```python
from build123d import *

# Parameters (mm, degrees)
BOSS_EXTRUDE1_DEPTH                   = 3.175
F_10_0_1935_DIAMETER_HOLE1_AT_2_COUNT = 2
F_10_0_1935_DIAMETER_HOLE1_AT_2_PITCH = 25.4
F_10_0_1935_DIAMETER_HOLE1_AT_3_COUNT = 2
F_10_0_1935_DIAMETER_HOLE1_AT_3_PITCH = 28.398063314
F_10_0_1935_DIAMETER_HOLE1_AT_4_COUNT = 2
F_10_0_1935_DIAMETER_HOLE1_AT_4_PITCH = 52.363441445


with BuildPart() as part:
    # Sketch2 → Boss-Extrude1 (new body)
    with BuildSketch(Plane(origin=(0, 0, 0), x_dir=(1, 0, 0), z_dir=(0, 1, 0))):
        Polygon((-0.378728756, 269.21115375), (50.421271244, 269.21115375), (50.421271244, 243.81115375), (37.721271244, 193.01115375), (12.321271244, 193.01115375), (-0.378728756, 243.81115375), align=None)
    extrude(amount=BOSS_EXTRUDE1_DEPTH)

    # Sketch7 → #10 (0.1935) Diameter Hole1 (revolve, cut)
    with BuildSketch(Plane(origin=(37.721271244, 0, -256.51115375), x_dir=(0, 0, -1), z_dir=(1, 0, 0))):
        Polygon((0, 0), (0, 3.175), (2.45745, 3.175), (2.45745, 3.177605133), (5.2197, 0), align=None)
    f_10_0_1935_diameter_hole1 = revolve(axis=Axis((37.721271244, -6.35, -256.51115375), (0, 1, 0)), mode=Mode.SUBTRACT)

    # #10 (0.1935) Diameter Hole1 at 2: #10 (0.1935) Diameter Hole1 ×2
    with Locations(*[(-i * F_10_0_1935_DIAMETER_HOLE1_AT_2_PITCH, 0, 0) for i in range(1, F_10_0_1935_DIAMETER_HOLE1_AT_2_COUNT)]):
        add(f_10_0_1935_diameter_hole1, mode=Mode.SUBTRACT)

    # #10 (0.1935) Diameter Hole1 at 3: #10 (0.1935) Diameter Hole1 ×2
    with Locations(*[Vector(-0.44721359549995443, 0, 0.8944271909999176) * (i * F_10_0_1935_DIAMETER_HOLE1_AT_3_PITCH) for i in range(1, F_10_0_1935_DIAMETER_HOLE1_AT_3_COUNT)]):
        add(f_10_0_1935_diameter_hole1, mode=Mode.SUBTRACT)

    # #10 (0.1935) Diameter Hole1 at 4: #10 (0.1935) Diameter Hole1 ×2
    with Locations(*[Vector(-0.24253562503633175, 0, 0.9701425001453322) * (i * F_10_0_1935_DIAMETER_HOLE1_AT_4_PITCH) for i in range(1, F_10_0_1935_DIAMETER_HOLE1_AT_4_COUNT)]):
        add(f_10_0_1935_diameter_hole1, mode=Mode.SUBTRACT)


solid = part.part
```
Geometry check sheet. Reference: the model listing, model coordinates, mm. Give positions to 0.01 mm unless a question says otherwise; leave off trailing zeros. Loops run counter-clockwise (first coordinate to the right, second up) from the corner with the lowest first, then second, coordinate; pieces in that order, holes last. Notation, with made-up numbers: M -23,-38 L 20,-38 A31 ccw 20,-4 Z; hole C 53.25,83.5 d10. An arc over 180 degrees is marked long. Answer as CSV lines item,"result".
Item 1: Release check for a two-part mould opening along X. For faces 1 (the flat face through (6.06, 1.57, -218.06)), 2 (the conical face through (26.03, 2.98, -233.54)), 3 (the conical face through (36.93, 2.98, -259.02)), 4 (the flat face through (25, 2, -269.211)) record: pulls with the +X half, pulls with the -X half, needs draft (parallel to the pull), parting line crosses it, or undercut.
Values:
face 1,"pulls with the -X half"
face 2,"undercut"
face 3,"undercut"
face 4,"needs draft"
Item 2: Depth check by flat-ended pin: P1, Ø1.5, axis at x = 18, z = -205.5, coming from the -Y side; P2, Ø5, axis at x = 13, z = -259, coming from the -Y side. Enter the tip coordinate at first touch or a pass-through.
Values:
P1,"stops at y = 0"
P2,"stops at y = 0.16"
Item 3: Cross-section at D-D on x = 47.5. Record the cut outline in (y, z) (3 decimals), and give its area (3 significant figures).
Values:
outline,"M 0,-269.211 L 3.175,-269.211 L 3.175,-232.126 L 0,-232.126 Z"
area,"118 mm²"
Item 4: Cross-section at C-C on z = -224. Record the cut outline in (x, y) (3 decimals), and give its area (3 significant figures).
Values:
outline,"M 4.574,0 L 45.468,0 L 45.468,3.175 L 4.574,3.175 Z"
area,"130 mm²"
Item 5: Material ranges on line 1 (X direction, y = 1.6, z = -258); line 2 (Z direction, x = 25, y = 1.4); line 3 (X direction, y = 0.7, z = -208), recorded low to high.
Values:
line 1,"x = -0.38 to 8.79, 15.85 to 34.19, 41.25 to 50.42"
line 2,"z = -269.21 to -235.11, -227.11 to -209.71, -201.71 to -193.01"
line 3,"x = 8.57 to 21.02, 29.02 to 41.47"
Item 6: Cross-section at B-B on x = 24. Count the separate pieces of the cut face and the enclosed holes in it, and give its area (3 significant figures).
Values:
separate pieces,"3"
enclosed holes,"0"
area,"195 mm²"
Item 7: Cross-section at A-A on y = 1.55. Record the cut outline in (x, z), and give its area (3 significant figures).
Values:
outline,"M -0.38,-269.21 L 50.42,-269.21 L 50.42,-243.81 L 37.72,-193.01 L 12.32,-193.01 L -0.38,-243.81 Z; hole C 12.32,-256.51 d7.74; hole C 25.02,-231.11 d7.74; hole C 25.02,-205.71 d7.74; hole C 37.72,-256.51 d7.74"
area,"3,040 mm²"
